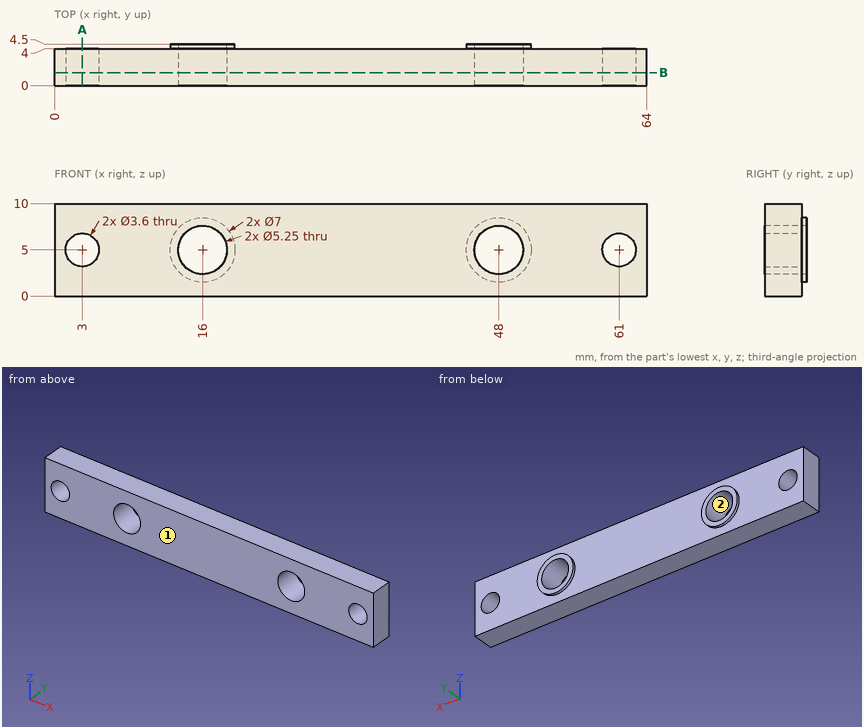
Source: three-view drawing plus pictorial views. Frame: mm from the lowest corner of the part. Round coordinates to 2 decimals unless told otherwise and drop trailing zeros. Order: outer loops, then holes, each group sorted by start corner. A loop starts at its lowest first (then second) coordinate and runs counter-clockwise, first axis right, second up. Notation, with made-up numbers: (67.25, 50) - (82.25, 50) arc R16 cw to (82.25, 66) - close; hole circle Ø1 at (0, 77). An arc over 180 degrees is marked (long way). Answer in a Markdown table with one row per item.
Item 1: Line query: line 1 (X direction, y = 3.2, z = 5) (3 decimals); line 2 (Z direction, x = 48, y = 2.6) (3 decimals); line 3 (X direction, y = 1.9, z = 7). Output: solid intervals per line, ascending.
Model answer:
| item | result |
|---|---|
| line 1 | x = 0 to 1.2, 4.8 to 13.375, 18.625 to 45.375, 50.625 to 59.2, 62.8 to 64 |
| line 2 | z = 0 to 2.375, 7.625 to 10 |
| line 3 | x = 0 to 14.3, 17.7 to 46.3, 49.7 to 64 |
Item 2: Mould query, pull axis X, two halves, no side actions, for the marked faces 1 and 2. Classes: released by +X, released by -X, zero draft, split by the parting line, or undercut.
Model answer:
| item | result |
|---|---|
| face 1 | zero draft |
| face 2 | undercut |
Item 3: Section query B-B (y = 1.4). Return the cut outline in (x, z) (3 decimals).
Model answer:
| item | result |
|---|---|
| outline | (0, 0) - (64, 0) - (64, 10) - (0, 10) - close; hole circle Ø3.6 at (3, 5); hole circle Ø5.25 at (16, 5); hole circle Ø5.25 at (48, 5); hole circle Ø3.6 at (61, 5) |
Item 4: Section query A-A (x = 3). Return the cut outline in (y, z).
Model answer:
| item | result |
|---|---|
| outline | (0, 0) - (4, 0) - (4, 3.2) - (0, 3.2) - close; (0, 6.8) - (4, 6.8) - (4, 10) - (0, 10) - close |
Item 5: Pin query (flat end, axial travel): pin 1 (4 mm diameter, centred on x = 61, z = 5, fed in from +Y); pin 2 (3 mm diameter, centred on x = 3, z = 5, fed in from -Y). Return the tip coordinate at first contact, or that it passes through.
Model answer:
| item | result |
|---|---|
| pin 1 | stops at y = 4 |
| pin 2 | passes through |
